```python
from build123d import *

# Parameters (mm, degrees)
F1_DEPTH = 12.7
F2_R     = 6.3065615495
F3_DEPTH = 12.7


with BuildPart() as f1:
    # F0 (on Front) → F1 (new body)
    with BuildSketch(Plane.XZ):
        with BuildLine():
            ThreePointArc((75.1826392346, -12.4101070791), (75.9452339179, -6.2258690285), (76.2, 0))
            ThreePointArc((76.2, 0), (75.9452339179, 6.2258690285), (75.1826392346, 12.4101070791))
            ThreePointArc((75.1826392346, 12.4101070791), (72.4705065417, 23.5470949714), (68.1185107432, 34.1512590416))
            ThreePointArc((68.1185107432, 34.1512590416), (61.6470949714, 44.7892362247), (53.5295549023, 54.2312340995))
            ThreePointArc((53.5295549023, 54.2312340995), (44.7892362247, 61.6470949714), (35.0354264109, 67.6680049669))
            ThreePointArc((35.0354264109, 67.6680049669), (23.5470949714, 72.4705065417), (11.43, 75.3378729458))
            Line((11.43, 75.3378729458), (-11.43, 75.3378729458))
            ThreePointArc((-11.43, 75.3378729458), (-23.5470949714, 72.4705065417), (-35.0354264109, 67.6680049669))
            ThreePointArc((-35.0354264109, 67.6680049669), (-44.7892362247, 61.6470949714), (-53.5295549023, 54.2312340995))
            ThreePointArc((-53.5295549023, 54.2312340995), (-61.6470949714, 44.7892362247), (-68.1185107432, 34.1512590416))
            ThreePointArc((-68.1185107432, 34.1512590416), (-72.4705065417, 23.5470949714), (-75.1826392346, 12.4101070791))
            ThreePointArc((-75.1826392346, 12.4101070791), (-76.2, 0), (-75.1826392346, -12.4101070791))
            ThreePointArc((-75.1826392346, -12.4101070791), (-72.4705065417, -23.5470949714), (-68.1185107432, -34.1512590416))
            ThreePointArc((-68.1185107432, -34.1512590416), (-61.6470949714, -44.7892362247), (-53.5295549023, -54.2312340995))
            ThreePointArc((-53.5295549023, -54.2312340995), (-44.7892362247, -61.6470949714), (-35.0354264109, -67.6680049669))
            ThreePointArc((-35.0354264109, -67.6680049669), (-23.5470949714, -72.4705065417), (-11.43, -75.3378729458))
            ThreePointArc((-11.43, -75.3378729458), (0, -76.2), (11.43, -75.3378729458))
            ThreePointArc((11.43, -75.3378729458), (23.5470949714, -72.4705065417), (35.0354264109, -67.6680049669))
            ThreePointArc((35.0354264109, -67.6680049669), (44.7892362247, -61.6470949714), (53.5295549023, -54.2312340995))
            ThreePointArc((53.5295549023, -54.2312340995), (61.6470949714, -44.7892362247), (68.1185107432, -34.1512590416))
            ThreePointArc((68.1185107432, -34.1512590416), (72.4705065417, -23.5470949714), (75.1826392346, -12.4101070791))
        make_face()
        with BuildLine():
            ThreePointArc((68.1185107432, 34.1512590416), (72.4705065417, 23.5470949714), (75.1826392346, 12.4101070791))
            Line((75.1826392346, 12.4101070791), (84.8453734402, 15.5497197419))
            Line((84.8453734402, 15.5497197419), (77.7812449488, 37.2908717044))
            Line((77.7812449488, 37.2908717044), (68.1185107432, 34.1512590416))
        make_face()
        with BuildLine():
            Line((84.8453734402, -15.5497197419), (75.1826392346, -12.4101070791))
            ThreePointArc((75.1826392346, -12.4101070791), (72.4705065417, -23.5470949714), (68.1185107432, -34.1512590416))
            Line((68.1185107432, -34.1512590416), (77.7812449488, -37.2908717044))
            Line((77.7812449488, -37.2908717044), (84.8453734402, -15.5497197419))
        make_face()
        with BuildLine():
            ThreePointArc((35.0354264109, 67.6680049669), (44.7892362247, 61.6470949714), (53.5295549023, 54.2312340995))
            Line((53.5295549023, 54.2312340995), (59.5014530656, 62.4508467624))
            Line((59.5014530656, 62.4508467624), (41.0073245742, 75.8876176298))
            Line((41.0073245742, 75.8876176298), (35.0354264109, 67.6680049669))
        make_face()
        with BuildLine():
            Line((59.5014530656, -62.4508467624), (53.5295549023, -54.2312340995))
            ThreePointArc((53.5295549023, -54.2312340995), (44.7892362247, -61.6470949714), (35.0354264109, -67.6680049669))
            Line((35.0354264109, -67.6680049669), (41.0073245742, -75.8876176298))
            Line((41.0073245742, -75.8876176298), (59.5014530656, -62.4508467624))
        make_face()
        with BuildLine():
            Line((-11.43, 75.3378729458), (11.43, 75.3378729458))
            ThreePointArc((11.43, 75.3378729458), (0, 76.2), (-11.43, 75.3378729458))
        make_face()
        with BuildLine():
            ThreePointArc((-11.43, 75.3378729458), (0, 76.2), (11.43, 75.3378729458))
            Line((11.43, 75.3378729458), (11.43, 85.4978729458))
            Line((11.43, 85.4978729458), (-11.43, 85.4978729458))
            Line((-11.43, 85.4978729458), (-11.43, 75.3378729458))
        make_face()
        with BuildLine():
            Line((11.43, -85.4978729458), (11.43, -75.3378729458))
            ThreePointArc((11.43, -75.3378729458), (0, -76.2), (-11.43, -75.3378729458))
            Line((-11.43, -75.3378729458), (-11.43, -85.4978729458))
            Line((-11.43, -85.4978729458), (11.43, -85.4978729458))
        make_face()
        with BuildLine():
            ThreePointArc((-53.5295549023, 54.2312340995), (-44.7892362247, 61.6470949714), (-35.0354264109, 67.6680049669))
            Line((-35.0354264109, 67.6680049669), (-41.0073245742, 75.8876176298))
            Line((-41.0073245742, 75.8876176298), (-59.5014530656, 62.4508467624))
            Line((-59.5014530656, 62.4508467624), (-53.5295549023, 54.2312340995))
        make_face()
        with BuildLine():
            Line((-41.0073245742, -75.8876176298), (-35.0354264109, -67.6680049669))
            ThreePointArc((-35.0354264109, -67.6680049669), (-44.7892362247, -61.6470949714), (-53.5295549023, -54.2312340995))
            Line((-53.5295549023, -54.2312340995), (-59.5014530656, -62.4508467624))
            Line((-59.5014530656, -62.4508467624), (-41.0073245742, -75.8876176298))
        make_face()
        with BuildLine():
            ThreePointArc((-75.1826392346, 12.4101070791), (-72.4705065417, 23.5470949714), (-68.1185107432, 34.1512590416))
            Line((-68.1185107432, 34.1512590416), (-77.7812449488, 37.2908717044))
            Line((-77.7812449488, 37.2908717044), (-84.8453734402, 15.5497197419))
            Line((-84.8453734402, 15.5497197419), (-75.1826392346, 12.4101070791))
        make_face()
        with BuildLine():
            Line((-77.7812449488, -37.2908717044), (-68.1185107432, -34.1512590416))
            ThreePointArc((-68.1185107432, -34.1512590416), (-72.4705065417, -23.5470949714), (-75.1826392346, -12.4101070791))
            Line((-75.1826392346, -12.4101070791), (-84.8453734402, -15.5497197419))
            Line((-84.8453734402, -15.5497197419), (-77.7812449488, -37.2908717044))
        make_face()
    extrude(amount=F1_DEPTH)

    # F2 (on face) → F3 (cut)
    with BuildSketch(Plane.XZ.offset(12.7)):
        Circle(F2_R)
    extrude(amount=-F3_DEPTH, mode=Mode.SUBTRACT)


solid = f1.part
```
Verification items for the finished model (mm, model axes). A direction names the side the tool comes from. Give positions to 0.01 mm unless a question says otherwise; leave off trailing zeros. Loops run counter-clockwise (first coordinate to the right, second up) from the corner with the lowest first, then second, coordinate; pieces in that order, holes last.
1. Go/stop test with flat-tipped pins: pin 1 Ø5 at (y, z) = (-4, -18.5) entering from +X; pin 2 Ø3 at (y, z) = (-3.5, 81) entering from +X; pin 3 Ø5 at (y, z) = (-4.5, 58) entering from -X. Record where each tip stops, or that it passes through.
2. Section check C-C, the plane z = -72. Enter the section's corners in (x, y).
3. Section check B-B, the plane z = -3. Enter the section's corners in (x, y), then the cut area to 3 significant figures.
4. Section check D-D, the plane z = 31.5. Enter the section's corners in (x, y), then the cut area to 3 significant figures.
5. Thickness scan on line 1 (Z direction, x = 0, y = -3.5); line 2 (Z direction, x = 1.5, y = -7.5); line 3 (Z direction, x = 58.5, y = -8.5). Record the ranges inside material, lowest first.
6. Set-up check for faces 1 (the flat face through (37.98, -6.26, -71.72)), 2 (the flat face through (-80.08, -6.26, 14)), 3 (the flat face through (-37.98, -6.26, 71.72)), 4 (the flat face through (56.47, -6.26, 58.28)): record each of +Z, -Z, +X, -X, +Y, -Y from which the full face is reachable in a straight line by a thin tool's end or side.
7. Mould release check, pull along X, two halves, no side actions. Record for faces 5 (the flat face through (79.95, -6.26, 13.96)), 6 (the cylindrical face through (-76.2, -6.3, 0.2)), 7 (the cylindrical face through (23.381, -6.261, -72.524)): released by +X, released by -X, zero draft, split by the parting line, or undercut.
8. Section check A-A, the plane x = 0. Enter the section's corners in (y, z), then the cut area to 3 significant figures.
Geometry says:
1. pin 1: stops at x = 84.7
1. pin 2: stops at x = 11.43
1. pin 3: stops at x = -58.08
2. outline: (-46.36, -12.7) - (-38.18, -12.7) - (-38.18, 0) - (-46.36, 0) - close; (-24.95, -12.7) - (24.95, -12.7) - (24.95, 0) - (-24.95, 0) - close; (38.18, -12.7) - (46.36, -12.7) - (46.36, 0) - (38.18, 0) - close
3. outline: (-76.14, -12.7) - (-5.55, -12.7) - (-5.55, 0) - (-76.14, 0) - close; (5.55, -12.7) - (76.14, -12.7) - (76.14, 0) - (5.55, 0) - close
3. area: 1,790 mm2
4. outline: (-79.66, -12.7) - (79.66, -12.7) - (79.66, 0) - (-79.66, 0) - close
4. area: 2,020 mm2
5. line 1: z = -85.5 to -6.31, 6.31 to 85.5
5. line 2: z = -85.5 to -6.13, 6.13 to 85.5
5. line 3: z = -63.18 to -61.07, -48.83 to 48.83, 61.07 to 63.18
6. face 1: -Z, +Y, -Y
6. face 2: -X, +Y, -Y
6. face 3: +Z, +Y, -Y
6. face 4: +X, +Y, -Y
7. face 5: released by +X
7. face 6: released by -X
7. face 7: undercut
8. outline: (-12.7, -85.5) - (0, -85.5) - (0, -6.31) - (-12.7, -6.31) - close; (-12.7, 6.31) - (0, 6.31) - (0, 85.5) - (-12.7, 85.5) - close
8. area: 2,010 mm2
